from build123d import *

# Parameters (mm, degrees)
BASE_DEPTH             = 16.1
SHELL_T                = -2
SCREEN_START           = 0.4
SCREEN_BASE_DEPTH      = 0.4
SKETCH21_R             = 1.6
LEG_HOLES_DEPTH        = 182.359773103
SCREEN_CLAMPS_DEPTH    = 0.4
SCREEN_CLAMP_FILLETS_R = 1
SKETCH23_R             = 1.35
CUT_EXTRUDE1_DEPTH     = 0.4
CUT_EXTRUDE2_DEPTH     = 191.280496373


with BuildPart() as part:
    # Sketch2 → Base (new body)
    with BuildSketch(Plane(origin=(0, 0, 0), x_dir=(1, 0, 0), z_dir=(0, 1, 0))):
        with BuildLine():
            Line((2.5, 0), (68, 0))
            ThreePointArc((68, 0), (69.767766953, 0.732233047), (70.5, 2.5))
            Line((70.5, 2.5), (70.5, 97.5))
            ThreePointArc((70.5, 97.5), (69.767766953, 99.267766953), (68, 100))
            Line((68, 100), (2.5, 100))
            ThreePointArc((2.5, 100), (0.732233047, 99.267766953), (0, 97.5))
            Line((0, 97.5), (0, 2.5))
            ThreePointArc((0, 2.5), (0.732233047, 0.732233047), (2.5, 0))
        make_face()
    extrude(amount=BASE_DEPTH)

    # Shell
    shell_openings = [part.faces().sort_by_distance(p)[0] for p in [
        (35.25, 16.1, -50),
        (35.25, 0, -50),
    ]]
    offset(amount=SHELL_T, openings=shell_openings, kind=Kind.INTERSECTION)

    # Sketch19 → Screen Base (add)
    with BuildSketch(Plane.XZ.offset(SCREEN_START)):
        with BuildLine():
            Line((-6.55, 46.74), (92.45, 46.74))
            ThreePointArc((92.45, 46.74), (98.022001436, 44.432001436), (100.33, 38.86))
            Line((100.33, 38.86), (100.33, -142.34))
            ThreePointArc((100.33, -142.34), (98.022001436, -147.912001436), (92.45, -150.22))
            Line((92.45, -150.22), (-6.55, -150.22))
            ThreePointArc((-6.55, -150.22), (-12.122001436, -147.912001436), (-14.43, -142.34))
            Line((-14.43, -142.34), (-14.43, 38.86))
            ThreePointArc((-14.43, 38.86), (-12.122001436, 44.432001436), (-6.55, 46.74))
        make_face()
        with BuildLine():
            Line((2.5, -98), (68, -98))
            ThreePointArc((68, -98), (68.353553391, -97.853553391), (68.5, -97.5))
            Line((68.5, -97.5), (68.5, -2.5))
            ThreePointArc((68.5, -2.5), (68.353553391, -2.146446609), (68, -2))
            Line((68, -2), (2.5, -2))
            ThreePointArc((2.5, -2), (2.146446609, -2.146446609), (2, -2.5))
            Line((2, -2.5), (2, -97.5))
            ThreePointArc((2, -97.5), (2.146446609, -97.853553391), (2.5, -98))
        make_face(mode=Mode.SUBTRACT)
    extrude(amount=-SCREEN_BASE_DEPTH)

    # Sketch21 → Leg Holes (cut, through all)
    with BuildSketch(Plane(origin=(0, 0, 0), x_dir=(1, 0, 0), z_dir=(0, 1, 0))):
        with Locations(Location((9.15, 113.35, 0), (0, 0, 270))):
            Circle(SKETCH21_R)
        with Locations(Location((74.8, 113.35, 0), (0, 0, 270))):
            Circle(SKETCH21_R)
        with Locations(Location((74.8, -12.85, 0), (0, 0, 270))):
            Circle(SKETCH21_R)
        with Locations(Location((9.15, -12.85, 0), (0, 0, 270))):
            Circle(SKETCH21_R)
    extrude(amount=-LEG_HOLES_DEPTH, mode=Mode.SUBTRACT)

    # Sketch22 → Screen Clamps (add)
    with BuildSketch(Plane(origin=(0, 0, 0), x_dir=(1, 0, 0), z_dir=(0, 1, 0))):
        with BuildLine():
            Line((-5.55, 152.42), (-5.55, 150.22))
            Line((-5.55, 150.22), (2.95, 150.22))
            Line((2.95, 150.22), (2.95, 152.42))
            ThreePointArc((2.95, 152.42), (-1.3, 156.67), (-5.55, 152.42))
        make_face()
        with BuildLine():
            Line((82.95, 152.42), (82.95, 150.22))
            Line((82.95, 150.22), (91.45, 150.22))
            Line((91.45, 150.22), (91.45, 152.42))
            ThreePointArc((91.45, 152.42), (87.2, 156.67), (82.95, 152.42))
        make_face()
        with BuildLine():
            Line((-5.55, -48.94), (-5.55, -46.74))
            Line((-5.55, -46.74), (2.95, -46.74))
            Line((2.95, -46.74), (2.95, -48.94))
            ThreePointArc((2.95, -48.94), (-1.3, -53.19), (-5.55, -48.94))
        make_face()
        with BuildLine():
            Line((82.95, -48.94), (82.95, -46.74))
            Line((82.95, -46.74), (91.45, -46.74))
            Line((91.45, -46.74), (91.45, -48.94))
            ThreePointArc((91.45, -48.94), (87.2, -53.19), (82.95, -48.94))
        make_face()
        with BuildLine():
            Line((-14.43, 123.44), (-16.63, 123.44))
            ThreePointArc((-16.63, 123.44), (-20.88, 119.19), (-16.63, 114.94))
            Line((-16.63, 114.94), (-14.43, 114.94))
            Line((-14.43, 114.94), (-14.43, 123.44))
        make_face()
        with BuildLine():
            Line((-14.43, -11.46), (-16.63, -11.46))
            ThreePointArc((-16.63, -11.46), (-20.88, -15.71), (-16.63, -19.96))
            Line((-16.63, -19.96), (-14.43, -19.96))
            Line((-14.43, -19.96), (-14.43, -11.46))
        make_face()
        with BuildLine():
            Line((100.33, -11.46), (102.53, -11.46))
            ThreePointArc((102.53, -11.46), (106.78, -15.71), (102.53, -19.96))
            Line((102.53, -19.96), (100.33, -19.96))
            Line((100.33, -19.96), (100.33, -11.46))
        make_face()
        with BuildLine():
            Line((100.33, 123.44), (102.53, 123.44))
            ThreePointArc((102.53, 123.44), (106.78, 119.19), (102.53, 114.94))
            Line((102.53, 114.94), (100.33, 114.94))
            Line((100.33, 114.94), (100.33, 123.44))
        make_face()
    extrude(amount=-SCREEN_CLAMPS_DEPTH)

    # Screen Clamp Fillets
    screen_clamp_fillets_edges = [part.edges().sort_by_distance(p)[0] for p in [
        (-5.55, -0.2, -150.22),
        (2.95, -0.2, -150.22),
        (82.95, -0.2, -150.22),
        (91.45, -0.2, -150.22),
        (2.95, -0.2, 46.74),
        (-5.55, -0.2, 46.74),
        (91.45, -0.2, 46.74),
        (82.95, -0.2, 46.74),
        (-14.43, -0.2, -114.94),
        (-14.43, -0.2, -123.44),
        (-14.43, -0.2, 19.96),
        (-14.43, -0.2, 11.46),
        (100.33, -0.2, 11.46),
        (100.33, -0.2, 19.96),
        (100.33, -0.2, -123.44),
        (100.33, -0.2, -114.94),
    ]]
    fillet(screen_clamp_fillets_edges, radius=SCREEN_CLAMP_FILLETS_R - 0.0001)  # a hair under: the kernel refuses the full size

    # Sketch23 → Cut-Extrude1 (cut)
    with BuildSketch(Plane(origin=(0, -0.4, 0), x_dir=(1, 0, 0), z_dir=(0, 1, 0))):
        with Locations(Location((-1.3, 152.42, 0), (0, 0, 90))):
            Circle(SKETCH23_R)
        with Locations(Location((87.2, 152.42, 0), (0, 0, 90))):
            Circle(SKETCH23_R)
        with Locations(Location((-1.3, -48.94, 0), (0, 0, 90))):
            Circle(SKETCH23_R)
        with Locations(Location((87.2, -48.94, 0), (0, 0, 90))):
            Circle(SKETCH23_R)
        with Locations(Location((-16.63, 119.19, 0), (0, 0, 90))):
            Circle(SKETCH23_R)
        with Locations(Location((102.53, 119.19, 0), (0, 0, 90))):
            Circle(SKETCH23_R)
        with Locations(Location((102.53, -15.71, 0), (0, 0, 90))):
            Circle(SKETCH23_R)
        with Locations(Location((-16.63, -15.71, 0), (0, 0, 90))):
            Circle(SKETCH23_R)
    extrude(amount=CUT_EXTRUDE1_DEPTH, mode=Mode.SUBTRACT)

    # Sketch24 → Cut-Extrude2 (cut, through all)
    with BuildSketch(Plane(origin=(0, 0, 0), x_dir=(1, 0, 0), z_dir=(0, 1, 0))):
        with BuildLine():
            Line((-16.63, 114.94), (-15.43, 114.94))
            ThreePointArc((-15.43, 114.94), (-14.722893219, 114.647106781), (-14.43, 113.94))
            Line((-14.43, 113.94), (-14.43, -10.46))
            ThreePointArc((-14.43, -10.46), (-14.722893219, -11.167106781), (-15.43, -11.46))
            Line((-15.43, -11.46), (-16.63, -11.46))
            ThreePointArc((-16.63, -11.46), (-20.88, -15.71), (-16.63, -19.96))
            Line((-16.63, -19.96), (-15.43, -19.96))
            ThreePointArc((-15.43, -19.96), (-14.722893219, -20.252893219), (-14.43, -20.96))
            Line((-14.43, -20.96), (-14.43, -38.86))
            ThreePointArc((-14.43, -38.86), (-12.122001436, -44.432001436), (-6.55, -46.74))
            ThreePointArc((-6.55, -46.74), (-5.842893219, -47.032893219), (-5.55, -47.74))
            Line((-5.55, -47.74), (-5.55, -48.94))
            ThreePointArc((-5.55, -48.94), (-1.3, -53.19), (2.95, -48.94))
            Line((2.95, -48.94), (2.95, -47.74))
            ThreePointArc((2.95, -47.74), (3.242893219, -47.032893219), (3.95, -46.74))
            Line((3.95, -46.74), (81.95, -46.74))
            ThreePointArc((81.95, -46.74), (82.657106781, -47.032893219), (82.95, -47.74))
            Line((82.95, -47.74), (82.95, -48.94))
            ThreePointArc((82.95, -48.94), (87.2, -53.19), (91.45, -48.94))
            Line((91.45, -48.94), (91.45, -47.74))
            ThreePointArc((91.45, -47.74), (91.742893219, -47.032893219), (92.45, -46.74))
            ThreePointArc((92.45, -46.74), (98.022001436, -44.432001436), (100.33, -38.86))
            Line((100.33, -38.86), (100.33, -20.96))
            ThreePointArc((100.33, -20.96), (100.622893219, -20.252893219), (101.33, -19.96))
            Line((101.33, -19.96), (102.53, -19.96))
            ThreePointArc((102.53, -19.96), (106.78, -15.71), (102.53, -11.46))
            Line((102.53, -11.46), (101.33, -11.46))
            ThreePointArc((101.33, -11.46), (100.622893219, -11.167106781), (100.33, -10.46))
            Line((100.33, -10.46), (100.33, 113.94))
            ThreePointArc((100.33, 113.94), (100.622893219, 114.647106781), (101.33, 114.94))
            Line((101.33, 114.94), (102.53, 114.94))
            ThreePointArc((102.53, 114.94), (106.78, 119.19), (102.53, 123.44))
            Line((102.53, 123.44), (101.33, 123.44))
            ThreePointArc((101.33, 123.44), (100.622893219, 123.732893219), (100.33, 124.44))
            Line((100.33, 124.44), (100.33, 142.34))
            ThreePointArc((100.33, 142.34), (98.022001436, 147.912001436), (92.45, 150.22))
            ThreePointArc((92.45, 150.22), (91.742893219, 150.512893219), (91.45, 151.22))
            Line((91.45, 151.22), (91.45, 152.42))
            ThreePointArc((91.45, 152.42), (87.2, 156.67), (82.95, 152.42))
            Line((82.95, 152.42), (82.95, 151.22))
            ThreePointArc((82.95, 151.22), (82.657106781, 150.512893219), (81.95, 150.22))
            Line((81.95, 150.22), (3.95, 150.22))
            ThreePointArc((3.95, 150.22), (3.242893219, 150.512893219), (2.95, 151.22))
            Line((2.95, 151.22), (2.95, 152.42))
            ThreePointArc((2.95, 152.42), (-1.3, 156.67), (-5.55, 152.42))
            Line((-5.55, 152.42), (-5.55, 151.22))
            ThreePointArc((-5.55, 151.22), (-5.842893219, 150.512893219), (-6.55, 150.22))
            ThreePointArc((-6.55, 150.22), (-12.122001436, 147.912001436), (-14.43, 142.34))
            Line((-14.43, 142.34), (-14.43, 124.44))
            ThreePointArc((-14.43, 124.44), (-14.722893219, 123.732893219), (-15.43, 123.44))
            Line((-15.43, 123.44), (-16.63, 123.44))
            ThreePointArc((-16.63, 123.44), (-20.88, 119.19), (-16.63, 114.94))
        make_face()
    extrude(amount=CUT_EXTRUDE2_DEPTH, mode=Mode.SUBTRACT)


solid = part.part
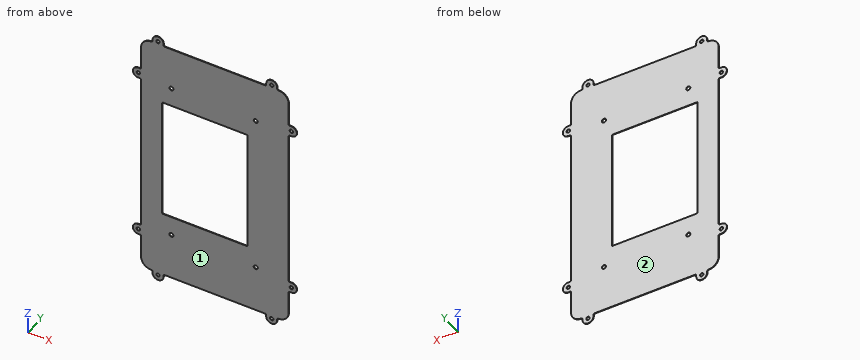
Can you work these out from the model? Positions are in its coordinate system, mm. Face numbers are marked on the shaded views. Round coordinates to 2 decimals unless told otherwise and drop trailing zeros. Write each loop counter-clockwise with the first axis right and the second up, starting at its lowest first coordinate (ties: lowest second). Pieces come first, ordered by that corner, then holes. Notation, with made-up numbers: (47, 76) -> (92, 76) arc R29 ccw to (92, 115) -> close; hole circle Ø1 at (58, -0.75). An arc over 180 degrees is marked (long way). Use one line per item in the form item = value. Start each with the question number.
Q1. Imagine slicing it at A-A (x = 46). Please give me the cut outline in (y, z), then the cut area to 3 significant figures.
Q2. We'd pull the mould along Y, two halves only. Please class the marked faces 1 and 2: +Y half, -Y half, draft (parallel to the pull), parting line (faces both ways), or undercut.
Q3. I'm going to push a flat-ended pin straight in: P1, Ø3, axis at x = -1.3, z = -152.42, coming from the +Y side. Where does the tip first touch, or does it pass through?
Q4. Imagine slicing it at B-B (y = -0.2). Count the separate pieces of the cut face and the enclosed holes in it, then the cut area to 3 significant figures.
Q5. If I drill on probe 1 along Z at (x, y) = (87.2, -0.2); probe 2 along X at (y, z) = (-0.25, -113.35); probe 3 along X at (y, z) = (-0.2, -119.19), over which ranges is the centre line in solid material (lowest first)? Write a range as [from, to].
Worked out:
q1.outline = (-0.4, -150.22) -> (0, -150.22) -> (0, -98) -> (-0.4, -98) -> close; (-0.4, -2) -> (0, -2) -> (0, 46.74) -> (-0.4, 46.74) -> close
q1.area = 40.4 mm^2
q2.face_1 = -Y half
q2.face_2 = +Y half
q3.P1 = 0
q4.separate_pieces = 1
q4.enclosed_holes = 13
q4.area = 16,500 mm^2
q5.probe_1 = [-156.67, -153.77], [-151.07, 47.59], [50.29, 53.19]
q5.probe_2 = [-14.43, 7.55], [10.75, 73.2], [76.4, 100.33]
q5.probe_3 = [-20.88, -17.98], [-15.28, 101.18], [103.88, 106.78]
